Part print with two shaded views. Sizes in mm from the minimum x, y, z corner. Round coordinates to 2 decimals unless told otherwise and drop trailing zeros. Write each loop counter-clockwise with the first axis right and the second up, starting at its lowest first coordinate (ties: lowest second). Pieces come first, ordered by that corner, then holes.
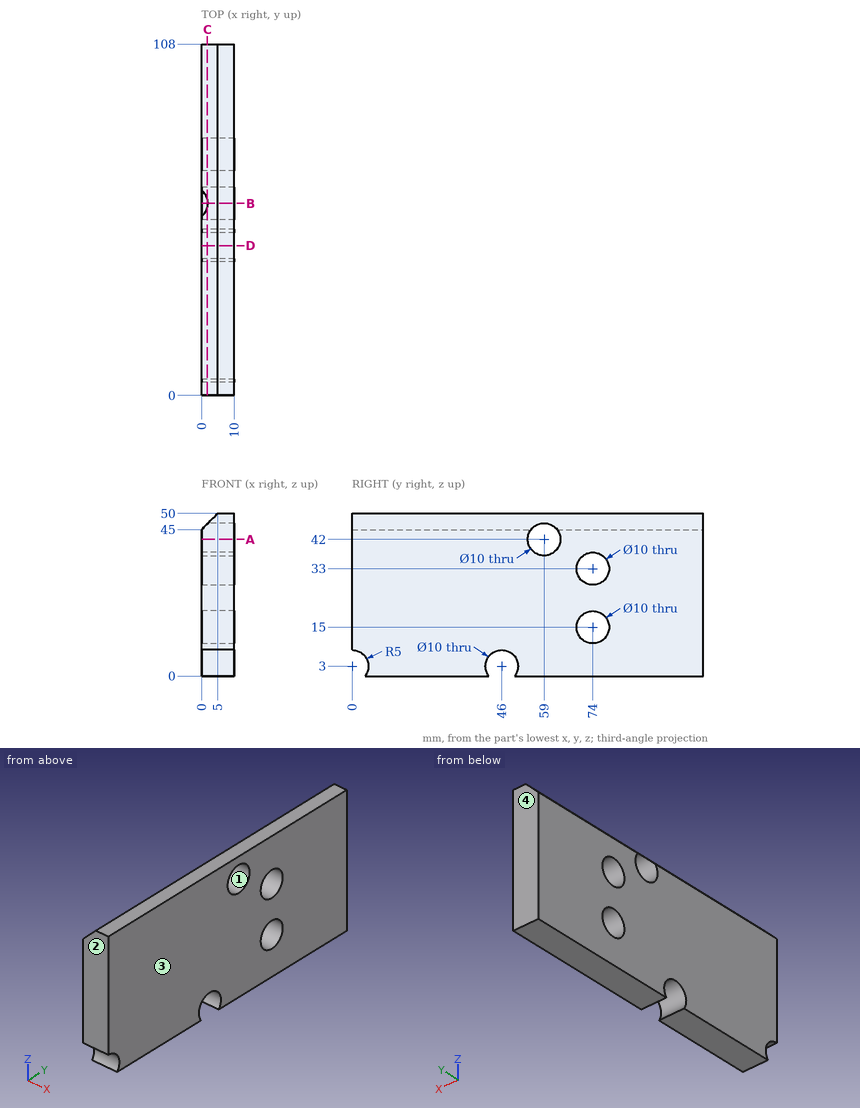
Q1. Drop flat-ended pins along their axis: pin 1 (6 mm diameter, centred on x = 4.5, z = 23.5, fed in from -Y); pin 2 (4 mm diameter, centred on x = 2, y = 38.5, fed in from +Z); pin 3 (6 mm diameter, centred on y = 74, z = 33, fed in from -X). Give the stop position or say it passes through.
Values follow:
pin 1: stops at y = 0
pin 2: stops at z = 49
pin 3: passes through
Q2. Cut at C-C on x = 1.75. Write the cut outline in (y, z).
Values follow:
outline: (0, 8) arc R5 cw to (4, 0) - (42, 0) arc R5 cw (long way) to (50, 0) - (108, 0) - (108, 46.75) - (60.56, 46.75) arc R5 cw (long way) to (57.44, 46.75) - (0, 46.75) - close; hole circle Ø10 at (74, 15); hole circle Ø10 at (74, 33)
Q3. Cut at D-D on y = 46. Write the cut outline in (x, z).
Values follow:
outline: (0, 8) - (10, 8) - (10, 50) - (5, 50) - (0, 45) - close
Q4. Cut at B-B on y = 59. Write the cut outline in (x, z), plus the area to 4 significant figures.
Values follow:
outline: (0, 0) - (10, 0) - (10, 37) - (0, 37) - close; (2, 47) - (10, 47) - (10, 50) - (5, 50) - close
area: 389.5 mm2
Q5. Wall check: L1, parallel to Z at x = 6.25, y = 74; L2, parallel to Y at x = 4.25, z = 15; L3, parallel to Y at x = 1, z = 37.5. Give the ranges that are in metal, low to high.
Values follow:
L1: z = 0 to 10, 20 to 28, 38 to 50
L2: y = 0 to 69, 79 to 108
L3: y = 0 to 56.82, 61.18 to 71.82, 76.18 to 108
Q6. Cut at A-A on z = 42. Write the cut outline in (x, y), plus the area to 3 significant figures.
Values follow:
outline: (0, 0) - (10, 0) - (10, 54) - (0, 54) - close; (0, 64) - (10, 64) - (10, 108) - (0, 108) - close
area: 980 mm2
Q7. Mould opens along Y. For the marked faces 1, 2, 3 and 4 say: +Y half, -Y half, draft (parallel to the pull), parting line (faces both ways), or undercut.
Values follow:
face 1: undercut
face 2: -Y half
face 3: draft
face 4: +Y half
